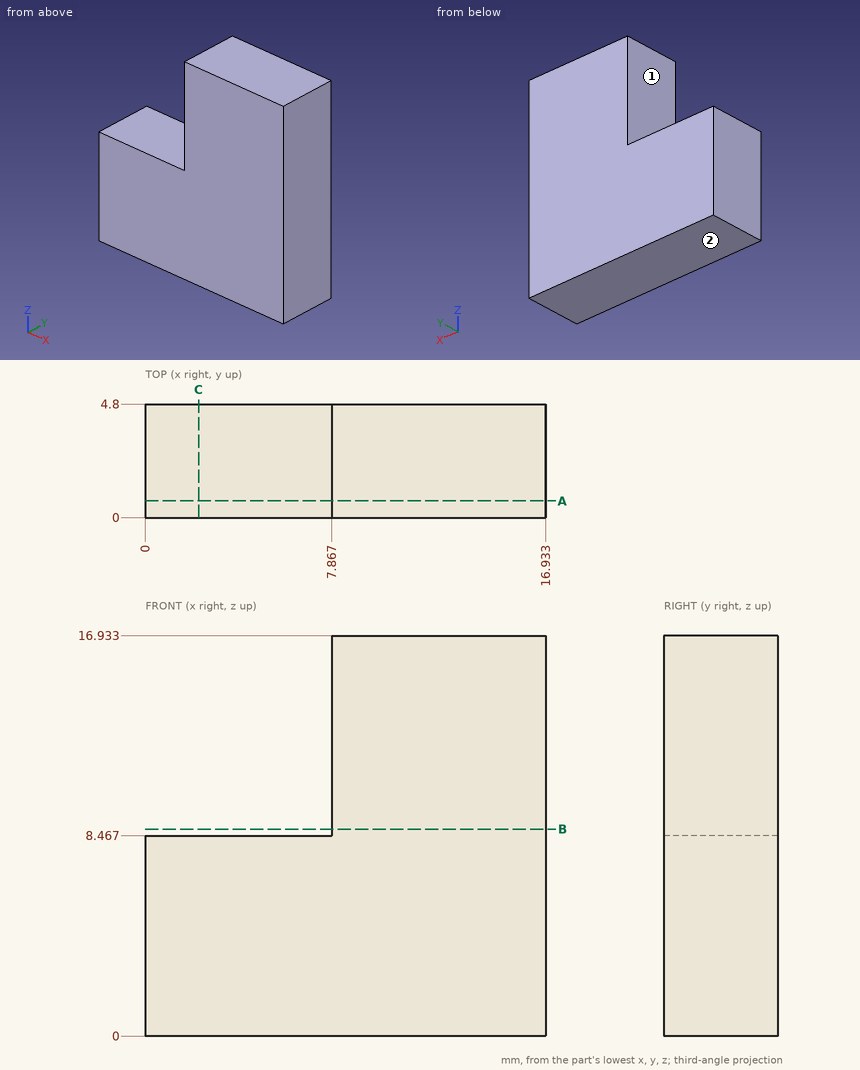
For this review, use the dimensioned drawing (mm, ordinates from the lowest corner) and the shaded views. A direction names the side the tool comes from. Give positions to 0.01 mm unless a question says otherwise; leave off trailing zeros. Loops run counter-clockwise (first coordinate to the right, second up) from the corner with the lowest first, then second, coordinate; pieces in that order, holes last.
Item 1: Take a section at A-A, the plane y = 0.7. State the section outline as (x, z) points, and give its area (3 significant figures).
Item 2: Take a section at B-B, the plane z = 8.75. State the section outline as (x, y) points.
Item 3: Tool access review of the marked faces 1 and 2: name each direction out of +Z, -Z, +X, -X, +Y, -Y from which nothing blocks a thin tool from reaching the whole face with its end or side.
Item 4: For line 1 along X through (y, z) = (3.1, 10.5); line 2 along Z through (x, y) = (2.75, 1.4), list the stretches that pass through material, from the lowest coordinate up.
Item 5: Take a section at C-C, the plane x = 2.25. State the section outline as (y, z) points.
Item 6: Insertion check: pin 1 (2.5 mm diameter, centred on y = 2.5, z = 11.5, fed in from -X). The pin has a flat end and moves straight along its axis. Give the tip position at first contact, or say it passes through.
Calculated:
1. outline: (0, 0) - (16.93, 0) - (16.93, 16.93) - (7.87, 16.93) - (7.87, 8.47) - (0, 8.47) - close
1. area: 220 mm2
2. outline: (7.87, 0) - (16.93, 0) - (16.93, 4.8) - (7.87, 4.8) - close
3. face 1: +Z, -X, +Y, -Y
3. face 2: -Z, +X, -X, +Y, -Y
4. line 1: x = 7.87 to 16.93
4. line 2: z = 0 to 8.47
5. outline: (0, 0) - (4.8, 0) - (4.8, 8.47) - (0, 8.47) - close
6. pin 1: stops at x = 7.87
